Model file for the job. Use its own axes, mm. Face numbers are marked on the shaded views. A direction names the side the tool comes from. Round coordinates to 2 decimals unless told otherwise and drop trailing zeros. Order: outer loops, then holes, each group sorted by start corner. A loop starts at its lowest first (then second) coordinate and runs counter-clockwise, first axis right, second up. Notation, with made-up numbers: (61, 71) -> (74, 71) arc R32 ccw to (74, 105) -> close; hole circle Ø7 at (4.25, 78.25). An arc over 180 degrees is marked (long way). Answer as CSV lines item,"result".
```python
from build123d import *

# Parameters (mm, degrees)
F0_R     = 25.4
F0_R_2   = 9.5885
F1_DEPTH = 9.525
F2_W     = 11.421807
F2_H     = 11.861946
F2_W_2   = 16.656801
F2_H_2   = 15.350755
F3_DEPTH = 17.78
F4_W     = 0.9144
F4_H     = 22.793547
F5_DEPTH = 15.5956
F6_R     = 9.7155
F7_DEPTH = 38.1


with BuildPart() as f1:
    # F0 (on Top) → F1 (new body, symmetric)
    with BuildSketch(Plane.XY):
        Circle(F0_R)
        Circle(F0_R_2, mode=Mode.SUBTRACT)
    extrude(amount=F1_DEPTH, both=True)

    # F2 (on Top) → F3 (cut, symmetric)
    with BuildSketch(Plane.XY):
        with Locations((-22.791632, -13.373764)):
            Rectangle(F2_W, F2_H)
        with Locations((28.368551, -15.118168)):
            Rectangle(F2_W_2, F2_H_2)
    extrude(amount=F3_DEPTH, both=True, mode=Mode.SUBTRACT)

    # F4 (on Top) → F5 (cut, symmetric)
    with BuildSketch(Plane.XY):
        with Locations((0, -17.44404)):
            Rectangle(F4_W, F4_H)
    extrude(amount=F5_DEPTH, both=True, mode=Mode.SUBTRACT)

    # F6 (on Top) → F7 (cut, symmetric)
    with BuildSketch(Plane.XY):
        Circle(F6_R)
    extrude(amount=F7_DEPTH, both=True, mode=Mode.SUBTRACT)


solid = f1.part
```
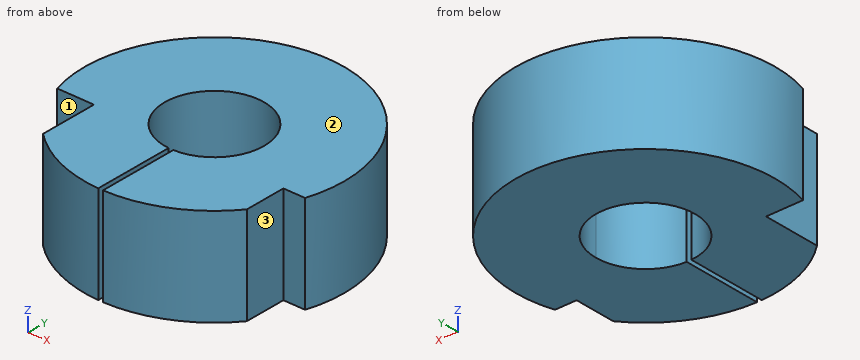
Q1. Wall check: L1, parallel to X at y = 0, z = 3.25; L2, parallel to X at y = -12.5, z = -5.25; L3, parallel to Y at x = 0, z = -0.75. Give the ranges that are in metal, low to high. Write a range as [from, to].
Checks:
L1,"[-25.4, -9.72], [9.72, 25.4]"
L2,"[-17.08, -0.46], [0.46, 20.04]"
L3,"[9.72, 25.4]"
Q2. Flat gauge pins, fed straight in: pin 1 (3.5 mm diameter, centred on y = -13, z = -1.5, fed in from -X); pin 2 (3.5 mm diameter, centred on x = 22.5, z = 0.5, fed in from -Y); pin 3 (6 mm diameter, centred on x = 15.5, z = -6, fed in from +Y). Where does each tip first touch, or does it go through?
Checks:
pin 1,"x = -17.08"
pin 2,"y = -7.44"
pin 3,"y = 22.11"
Q3. Saw through at A-A (z = -4.25). Write the cut outline in (x, y).
Checks:
outline,"(-24.29, -7.44) -> (-17.08, -7.44) -> (-17.08, -18.8) arc R25.4 ccw to (-0.46, -25.4) -> (-0.46, -9.7) arc R9.72 cw (long way) to (0.46, -9.7) -> (0.46, -25.4) arc R25.4 ccw to (20.04, -15.61) -> (20.04, -7.44) -> (24.29, -7.44) arc R25.4 ccw (long way) to start"
Q4. Tool access for the marked faces 1, 2 and 3: list every direction of +Z, -Z, +X, -X, +Y, -Y with a clear straight run to the whole face (end or side of a thin tool).
Checks:
face 1,"+Z, -Z, -X, -Y"
face 2,"+Z, +X, -X, +Y, -Y"
face 3,"+Z, -Z, +X, -Y"
Q5. Saw through at D-D (x = 15.5). Write the cut outline in (y, z) (3 decimals).
Checks:
outline,"(-20.122, -9.525) -> (20.122, -9.525) -> (20.122, 9.525) -> (-20.122, 9.525) -> close"
Q6. Saw through at C-C (y = -5). Write the cut outline in (x, z) (3 decimals), plus the area to 3 significant figures.
Checks:
outline,"(-24.903, -9.525) -> (-8.33, -9.525) -> (-8.33, 9.525) -> (-24.903, 9.525) -> close; (8.33, -9.525) -> (24.903, -9.525) -> (24.903, 9.525) -> (8.33, 9.525) -> close"
area,"631 mm²"
Q7. Saw through at B-B (x = -7). Write the cut outline in (y, z) (3 decimals).
Checks:
outline,"(-24.416, -9.525) -> (-6.737, -9.525) -> (-6.737, 9.525) -> (-24.416, 9.525) -> close; (6.737, -9.525) -> (24.416, -9.525) -> (24.416, 9.525) -> (6.737, 9.525) -> close"
